Study the drawing (mm; zero at the part's minimum x, y, z) and answer. A direction names the side the tool comes from. Give positions to 0.01 mm unless a question says otherwise; leave off trailing zeros. Order: outer loops, then holes, each group sorted by start corner. A loop starts at its lowest first (then second) coordinate and runs counter-clockwise, first axis right, second up.
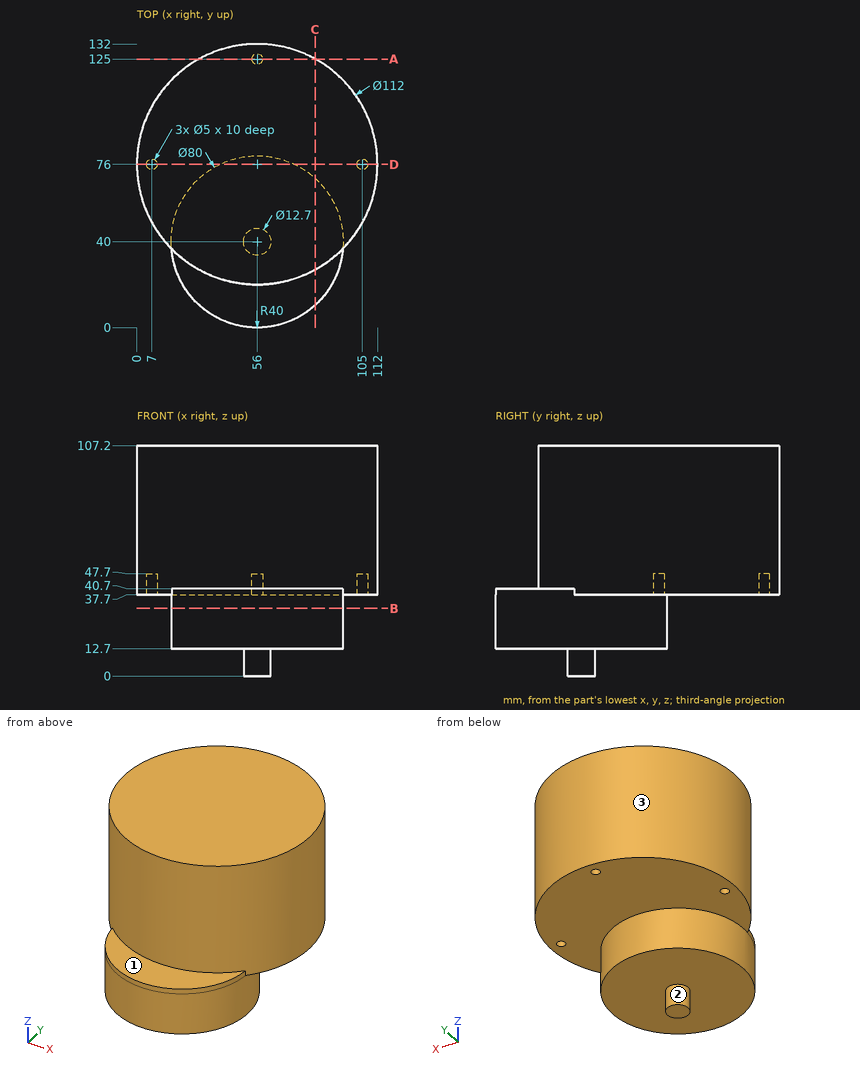
1) Find section A-A (y = 125). Write down the section's boundary in (x, z).
Geometry says:
outline: (28.89, 37.7) - (53.5, 37.7) - (53.5, 47.7) - (58.5, 47.7) - (58.5, 37.7) - (83.11, 37.7) - (83.11, 107.2) - (28.89, 107.2) - close
2) Find section C-C (x = 83). Write down the section's boundary in (y, z).
Geometry says:
outline: (10.49, 12.7) - (69.51, 12.7) - (69.51, 37.7) - (125.06, 37.7) - (125.06, 107.2) - (26.94, 107.2) - (26.94, 40.7) - (10.49, 40.7) - close
3) Given P1, Ø2.5, axis at x = 56, y = 124, coming from the -Z side; P2, Ø18.5, axis at x = 53.5, y = 17.5, coming from the +Z side; P3, Ø12, axis at y = 93, z = 51.5, coming from the -X side; P4, Ø5, axis at x = 25.5, z = 72, coming from the +Y side, each flat-ended and moving along its own axis, determine where each tip first touches the part or whether it passes through.
Geometry says:
P1: stops at z = 47.7
P2: stops at z = 107.2
P3: stops at x = 1.09
P4: stops at y = 124.5
4) Find section D-D (y = 76). Write down the section's boundary in (x, z).
Geometry says:
outline: (0, 37.7) - (4.5, 37.7) - (4.5, 47.7) - (9.5, 47.7) - (9.5, 37.7) - (38.56, 37.7) - (38.56, 12.7) - (73.44, 12.7) - (73.44, 37.7) - (102.5, 37.7) - (102.5, 47.7) - (107.5, 47.7) - (107.5, 37.7) - (112, 37.7) - (112, 107.2) - (0, 107.2) - close
5) A tool of negligible diameter and unlimited length cuts with its end or side. For the marked faces 1, 2 and 3, from which of +Z, -Z, +X, -X, +Y, -Y can it reach the whole face along a straight path? Write none if from no direction.
Geometry says:
face 1: +Z, -Y
face 2: -Z
face 3: +Z
6) Find section B-B (z = 31.5). Write down the section's boundary in (x, y).
Geometry says:
outline: circle Ø80 at (56, 40)
7) Straight lines are drawn through the part: probe 1 along Z at (x, y) = (74.5, 55.5); probe 2 along Y at (x, z) = (7, 40); probe 3 along Z at (x, y) = (27, 87.5). For each, find the intervals that lie inside material, in ascending order.
Geometry says:
probe 1: z = 12.7 to 107.2
probe 2: y = 48.89 to 73.5, 78.5 to 103.11
probe 3: z = 37.7 to 107.2
